```python
from build123d import *

# Parameters (mm, degrees)
SALIENTE_EXTRUIR1_DEPTH       = 75
CROQUIS2_R                    = 6.35
SALIENTE_EXTRUIR2_DEPTH       = 15
CORTAR_EXTRUIR1_DEPTH         = 85.541735255
CORTAR_EXTRUIR1_DEPTH_BACK    = 85.541735255
CORTAR_EXTRUIR2_DEPTH         = 85.541735255
CORTAR_EXTRUIR2_DEPTH_BACK    = 85.541735255
TALADRO_ROSCADO_1_4_201_D     = 5.1054
TALADRO_ROSCADO_1_4_201_DEPTH = 6.35


with BuildPart() as part:
    # Croquis1 → Saliente-Extruir1 (new, symmetric)
    with BuildSketch(Plane.XY):
        Polygon((0, 12.7), (0, -12.7), (25.4, -12.7), (25.4, -19.05), (-19.05, -19.05), (-19.05, 19.05), (25.4, 19.05), (25.4, 12.7), align=None)
    extrude(amount=SALIENTE_EXTRUIR1_DEPTH, both=True)

    # Croquis2 → Saliente-Extruir2 (add)
    with BuildSketch(Plane.ZY.offset(19.05)):
        with Locations(Location((-60, 0, 0), (0, 0, 180))):
            Circle(CROQUIS2_R)
    extrude(amount=SALIENTE_EXTRUIR2_DEPTH)

    # Croquis3 → Cortar-Extruir1 (cut, two sides: drawn at the far end of the back side and taken through both)
    with BuildSketch(Plane(origin=(0, 0, 0), x_dir=(1, 0, 0), z_dir=(0, 1, 0)).offset(-CORTAR_EXTRUIR1_DEPTH_BACK)):
        with BuildLine():
            Line((-4.525, -26), (-4.525, -56))
            ThreePointArc((-4.525, -56), (-9.525, -61), (-14.525, -56))
            Line((-14.525, -56), (-14.525, -26))
            ThreePointArc((-14.525, -26), (-9.525, -21), (-4.525, -26))
        make_face()
    extrude(amount=CORTAR_EXTRUIR1_DEPTH + CORTAR_EXTRUIR1_DEPTH_BACK, mode=Mode.SUBTRACT)

    # Croquis4 → Cortar-Extruir2 (cut, two sides: drawn at the far end of the back side and taken through both)
    with BuildSketch(Plane(origin=(0, 0, 0), x_dir=(0, 0, -1), z_dir=(1, 0, 0)).offset(-CORTAR_EXTRUIR2_DEPTH_BACK)):
        with BuildLine():
            ThreePointArc((-18.2012838, 6.841725806), (-18.5, 0), (-18.2012838, -6.841725806))
            ThreePointArc((-18.2012838, -6.841725806), (-14.409557257, -10.023362149), (-11.227920914, -6.231635606))
            ThreePointArc((-11.227920914, -6.231635606), (-11.5, 0), (-11.227920914, 6.231635606))
            ThreePointArc((-11.227920914, 6.231635606), (-14.409557257, 10.023362149), (-18.2012838, 6.841725806))
        make_face()
    extrude(amount=CORTAR_EXTRUIR2_DEPTH + CORTAR_EXTRUIR2_DEPTH_BACK, mode=Mode.SUBTRACT)

    # Taladro roscado 1/4-201
    with Locations(Plane(origin=(0, 19.05, 0), x_dir=(1, 0, 0), z_dir=(0, 1, 0))):
        with Locations((12.7, -50), (12.7, 50)):
            Hole(TALADRO_ROSCADO_1_4_201_D / 2, depth=TALADRO_ROSCADO_1_4_201_DEPTH)


solid = part.part
```
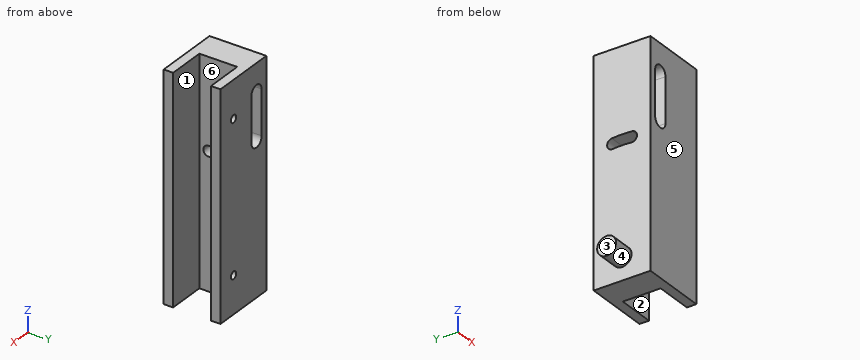
Geometry: final body of the model. Coordinates: model frame, mm. Face numbers are marked on the shaded views. A direction names the side the tool comes from. Round coordinates to 2 decimals unless told otherwise and drop trailing zeros. Order: outer loops, then holes, each group sorted by start corner. A loop starts at its lowest first (then second) coordinate and runs counter-clockwise, first axis right, second up. Notation, with made-up numbers: (87.5, 22) - (135.5, 22) arc R29 ccw to (135.5, 61) - close; hole circle Ø10 at (44, 88). An arc over 180 degrees is marked (long way). Write item = value, one per line. Start each with the question number.
Q1. Cut plane C-C on y = 0. Return the cut outline in (x, z) (3 decimals), and give its area (3 significant figures).
Q2. Pull-direction query (Y, two-part tool) for the marked faces 1, 2, 3 and 4; classes: +Y half, -Y half, draft (parallel to the pull), parting line (faces both ways), or undercut.
Q3. Cut plane D-D on x = 1.5. Return the cut outline in (y, z).
Q4. Pin query (flat end, axial travel): pin 1 (3 mm diameter, centred on x = 12.7, z = -50, fed in from +Y); pin 2 (7.5 mm diameter, centred on y = -4.5, z = 13.5, fed in from +X); pin 3 (9 mm diameter, centred on y = -1, z = 47.5, fed in from -X). Return the tip coordinate at first contact, or that it passes through.
Q5. Cut plane A-A on x = 12.7. Return the cut outline in (y, z), and give its area (3 significant figures).
Q6. Cut plane B-B on z = -50. Return the cut outline in (x, y), and give its area (3 significant figures).
Q7. Ray query, line 1 (X direction, y = 16.5, z = 50) (3 decimals); line 2 (Z direction, x = 12.7, y = 15); line 3 (Y direction, x = 19, z = -59). Return the intervals inside material, ascending. Write a range as from..to.
Q8. Access query for the marked faces 5 and 6. Directions: +Z, -Z, +X, -X, +Y, -Y. A direction counts if a zero-diameter tool reaches every point of the face in a straight line with its end or side. Return the directions, or none.
Outcome:
q1.outline = (-34.05, -66.35) - (-19.05, -66.35) - (-19.05, -75) - (0, -75) - (0, 11.5) - (-19.05, 11.5) - (-19.05, -53.65) - (-34.05, -53.65) - close; (-19.05, 18.5) - (0, 18.5) - (0, 75) - (-19.05, 75) - close; hole (-14.525, 26) arc R5 ccw to (-4.525, 26) - (-4.525, 56) arc R5 ccw to (-14.525, 56) - close
q1.area = 2,540 mm^2
q2.face_1 = undercut
q2.face_2 = undercut
q2.face_3 = draft
q2.face_4 = parting line
q3.outline = (-19.05, -75) - (-12.7, -75) - (-12.7, 75) - (-19.05, 75) - close; (12.7, -75) - (19.05, -75) - (19.05, 75) - (12.7, 75) - close
q4.pin_1 = -12.7
q4.pin_2 = 0
q4.pin_3 = -19.05
q5.outline = (-19.05, -75) - (-12.7, -75) - (-12.7, 75) - (-19.05, 75) - close; (12.7, -75) - (19.05, -75) - (19.05, -52.55) - (12.7, -52.55) - close; (12.7, -47.45) - (19.05, -47.45) - (19.05, 47.45) - (12.7, 47.45) - close; (12.7, 52.55) - (19.05, 52.55) - (19.05, 75) - (12.7, 75) - close
q5.area = 1,840 mm^2
q6.outline = (-19.05, -19.05) - (25.4, -19.05) - (25.4, -12.7) - (0, -12.7) - (0, 12.7) - (10.15, 12.7) - (10.15, 19.05) - (-19.05, 19.05) - close; (15.25, 12.7) - (25.4, 12.7) - (25.4, 19.05) - (15.25, 19.05) - close
q6.area = 1,020 mm^2
q7.line_1 = -19.05..-14.525, -4.525..10.147, 15.253..25.4
q7.line_2 = -75..-52.55, -47.45..47.45, 52.55..75
q7.line_3 = -19.05..-12.7, 12.7..19.05
q8.face_5 = +Z, -Z, +X, -X, -Y
q8.face_6 = +Z, -Z, +X
